Geometry: final body of the model. Coordinates: model frame, mm. A direction names the side the tool comes from. Give positions to 0.01 mm unless a question says otherwise; leave off trailing zeros. Loops run counter-clockwise (first coordinate to the right, second up) from the corner with the lowest first, then second, coordinate; pieces in that order, holes last.
1. Section C-C, the plane x = -110.75. Output: boundary loops of the cut face in (y, z).
2. First-contact query: P1, Ø2, axis at x = -121.5, z = 24, coming from the -Y side; P2, Ø3, axis at x = -114, y = 53, coming from the -Z side; P3, Ø3, axis at x = -121.5, z = 20.5, coming from the +Y side. Flat tips, straight axial feed; report the tip coordinate or a pass-through.
3. Access query for faces 4 (the face through (-114, 53, 10)), 5 (the face through (-125.46, 34.06, 19.72)). Directions: +Z, -Z, +X, -X, +Y, -Y. A direction counts if a zero-diameter tool reaches every point of the face in a straight line with its end or side. Return the directions, or none.
4. Section A-A, the plane z = 28. Output: boundary loops of the cut face in (x, y), then the cut area to 3 significant figures.
5. Material intervals for line 1 along Z through (x, y) = (-126, 11.5); line 2 along X through (y, z) = (3, 6); line 3 along X through (y, z) = (57, 31), sorted ascending.
6. Draft query along Y for faces 1 (the face through (-125, 0, 20)), 2 (the face through (-112.233, 63.781, 20.28)), 3 (the face through (-126.93, 11.54, 4.93)). Return one class per face: +Y half, -Y half, draft (parallel to the pull), parting line (faces both ways), or undercut.
7. Section D-D, the plane y = 40. Output: boundary loops of the cut face in (x, z), then the cut area to 3 significant figures.
8. Section B-B, the plane z = 9. Output: boundary loops of the cut face in (x, y).
from build123d import *

# Parameters (mm, degrees)
EXTRUDE_1_DEPTH     = 40
FILLET_1_R          = 3
SKETCH_2_R          = 2
CUT_EXTRUDE_1_DEPTH = 10


with BuildPart() as part:
    # 草图1 → 凸台-拉伸1 (new body)
    with BuildSketch(Plane.XY):
        with BuildLine():
            Line((-130, 0), (-120.5, 0))
            ThreePointArc((-120.5, 0), (-116.394062068, 31.187694935), (-104.356061156, 60.25))
            Line((-104.356061156, 60.25), (-112.583302492, 65))
            ThreePointArc((-112.583302492, 65), (-125.570357418, 33.646475863), (-130, 0))
        make_face()
    extrude(amount=EXTRUDE_1_DEPTH)

    # 圆角1
    fillet_1_edges = [part.edges().sort_by_distance(p)[0] for p in [
        (-104.356061156, 60.25, 20),
        (-120.5, 0, 20),
        (-130, 0, 20),
        (-112.583302492, 65, 20),
    ]]
    fillet(fillet_1_edges, radius=FILLET_1_R)

    # 草图2 → 切除-拉伸1 (cut)
    with BuildSketch(Plane(origin=(0, 0, 0), x_dir=(-1, 0, 0), z_dir=(0, 0, -1))):
        with Locations((125.022434611, 10.938045715)):
            Circle(SKETCH_2_R)
        with Locations((113.741627273, 53.038591848)):
            Circle(SKETCH_2_R)
    extrude(amount=-CUT_EXTRUDE_1_DEPTH, mode=Mode.SUBTRACT)


solid = part.part
Answers below:
1. outline: (47.48, 0) - (63.8, 0) - (63.8, 40) - (47.48, 40) - close
2. P1: stops at y = 0.16
2. P2: stops at z = 10
2. P3: stops at y = 50
3. face 4: -Z
3. face 5: +Z, -Z, -X, +Y
4. outline: (-129.96, 3.07) arc R3 ccw to (-126.96, 0) - (-123.46, 0) arc R3 ccw to (-120.46, 2.93) arc R120.5 cw to (-105.79, 57.7) arc R3 ccw to (-106.92, 61.73) - (-109.95, 63.48) arc R3 ccw to (-114.09, 62.32) arc R130 ccw to start
4. area: 615 mm2
5. line 1: z = 10 to 40
5. line 2: x = -129.96 to -120.46
5. line 3: x = -116.84 to -106.17
6. face 1: -Y half
6. face 2: +Y half
6. face 3: undercut
7. outline: (-123.69, 0) - (-113.67, 0) - (-113.67, 40) - (-123.69, 40) - close
7. area: 401 mm2
8. outline: (-129.96, 3.07) arc R3 ccw to (-126.96, 0) - (-123.46, 0) arc R3 ccw to (-120.46, 2.93) arc R120.5 cw to (-105.79, 57.7) arc R3 ccw to (-106.92, 61.73) - (-109.95, 63.48) arc R3 ccw to (-114.09, 62.32) arc R130 ccw to start; hole circle Ø4 at (-125.02, 10.94); hole circle Ø4 at (-113.74, 53.04)
